The figure shows three views and two pictorial views of one solid part (mm, origin at its lowest corner). Answer the questions. A direction names the side the tool comes from. Round coordinates to 2 decimals unless told otherwise and drop trailing zeros. Write each loop counter-clockwise with the first axis right and the second up, starting at its lowest first coordinate (ties: lowest second). Pieces come first, ordered by that corner, then holes. Notation, with made-up numbers: (89, 53) -> (133, 53) arc R15 ccw to (133, 75) -> close; hole circle Ø7 at (12.25, 16). An arc over 180 degrees is marked (long way). One line per item, written item: value.
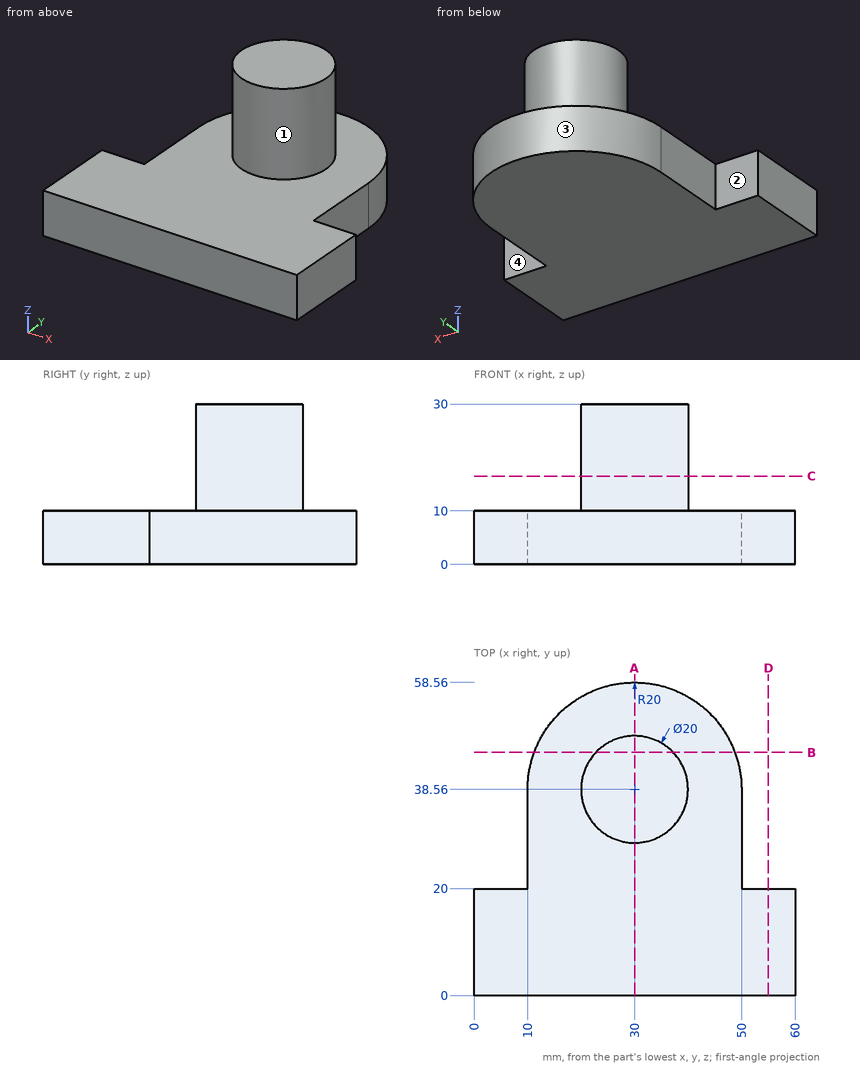
(1) Consider probe 1 along Y at (x, z) = (5, 4.75); probe 2 along Z at (x, y) = (44.5, 38.5); probe 3 along X at (y, z) = (21.5, 3.5). Determine where each line is inside the solid, lowest interval first.
Reported:
probe 1: y = 0 to 20
probe 2: z = 0 to 10
probe 3: x = 10 to 50
(2) Find section B-B on y = 45.5. Give the vertices of the cut face in (x, z), plus the area to 3 significant figures.
Reported:
outline: (11.24, 0) -> (48.76, 0) -> (48.76, 10) -> (37.2, 10) -> (37.2, 30) -> (22.8, 30) -> (22.8, 10) -> (11.24, 10) -> close
area: 663 mm2
(3) Find section D-D on x = 55. Give the vertices of the cut face in (y, z), plus the area to 3 significant figures.
Reported:
outline: (0, 0) -> (20, 0) -> (20, 10) -> (0, 10) -> close
area: 200 mm2
(4) A tool of negligible diameter and unlimited length cuts with its end or side. For the marked faces 1, 2, 3 and 4, from which of +Z, -Z, +X, -X, +Y, -Y can it reach the whole face along a straight path? Write none if from no direction.
Reported:
face 1: +Z
face 2: +Z, -Z, -X, +Y
face 3: +Z, -Z, +Y
face 4: +Z, -Z, +X, +Y
(5) Find section A-A on x = 30. Give the vertices of the cut face in (y, z).
Reported:
outline: (0, 0) -> (58.56, 0) -> (58.56, 10) -> (48.56, 10) -> (48.56, 30) -> (28.56, 30) -> (28.56, 10) -> (0, 10) -> close
(6) Flat-ended cylindrical pins translate along their axes: pin 1 Ø1.5 at (y, z) = (8, 11) entering from +X; pin 2 Ø6 at (y, z) = (44.5, 13.5) entering from -X; pin 3 Ø3 at (x, z) = (3.5, 5.5) entering from +Y; pin 4 Ø12 at (x, z) = (37.5, 10) entering from +Y. Find the tip coordinate at first contact, or state that the pin passes through.
Reported:
pin 1: passes through
pin 2: stops at x = 20.44
pin 3: stops at y = 20
pin 4: stops at y = 58.5
(7) Find section C-C on z = 16.5. Give the vertices of the cut face in (x, y).
Reported:
outline: circle Ø20 at (30, 38.56)
